from build123d import *

# Parameters (mm, degrees)
BOSS_EXTRUDE1_DEPTH = 6
SKETCH4_R           = 1
CUT_EXTRUDE2_DEPTH  = 230.888016217
SKETCH5_W           = 200
SKETCH5_H           = 20
BOSS_EXTRUDE2_DEPTH = 6
SKETCH6_W           = 184
SKETCH6_H           = 25
CUT_EXTRUDE3_DEPTH  = 230.888016217
SKETCH7_R           = 1
CUT_EXTRUDE4_DEPTH  = 6
BOSS_EXTRUDE3_DEPTH = 6
SKETCH9_R           = 1
CUT_EXTRUDE5_DEPTH  = 245.02561341
SKETCH10_W          = 15
SKETCH10_H          = 143.586884574
BOSS_EXTRUDE4_DEPTH = 6
SKETCH11_R          = 1
CUT_EXTRUDE6_DEPTH  = 245.02561341


with BuildPart() as part:
    # Sketch2 → Boss-Extrude1 (new body)
    with BuildSketch(Plane(origin=(0, 0, 0), x_dir=(1, 0, 0), z_dir=(0, 1, 0))):
        with BuildLine():
            Line((-100, -128.086884574), (-100, 35.5))
            Line((-100, 35.5), (100, 35.5))
            Line((100, 35.5), (100, -128.086884574))
            ThreePointArc((100, -128.086884574), (0, 162.5), (-100, -128.086884574))
        make_face()
    extrude(amount=BOSS_EXTRUDE1_DEPTH)

    # Sketch4 → Cut-Extrude2 (cut, through all)
    with BuildSketch(Plane(origin=(0, 6, 0), x_dir=(1, 0, 0), z_dir=(0, 1, 0))):
        with Locations(Location((119.15, -101.158131161, 0), (0, 0, 270))):
            Circle(SKETCH4_R)
        with Locations(Location((87.75, 86.5, 0), (0, 0, 270))):
            Circle(SKETCH4_R)
        with Locations(Location((152, 23.589123318, 0), (0, 0, 270))):
            Circle(SKETCH4_R)
        with Locations(Location((-87.75, 86.5, 0), (0, 0, 90))):
            Circle(SKETCH4_R)
        with Locations(Location((99, 36.6, 0), (0, 0, 270))):
            Circle(SKETCH4_R)
        with Locations(Location((-99, 36.6, 0), (0, 0, 90))):
            Circle(SKETCH4_R)
        with Locations(Location((-152, 23.589123318, 0), (0, 0, 90))):
            Circle(SKETCH4_R)
        with Locations(Location((-119.15, -101.158131161, 0), (0, 0, 90))):
            Circle(SKETCH4_R)
    extrude(amount=-CUT_EXTRUDE2_DEPTH, mode=Mode.SUBTRACT)

    # Sketch5 → Boss-Extrude2 (add)
    with BuildSketch(Plane(origin=(0, 6, 0), x_dir=(1, 0, 0), z_dir=(0, 1, 0))):
        with Locations((0, -118.086884574)):
            Rectangle(SKETCH5_W, SKETCH5_H)
    extrude(amount=-BOSS_EXTRUDE2_DEPTH)

    # Sketch6 → Cut-Extrude3 (cut, through all)
    with BuildSketch(Plane(origin=(0, 6, 0), x_dir=(1, 0, 0), z_dir=(0, 1, 0))):
        with Locations((0, 48)):
            Rectangle(SKETCH6_W, SKETCH6_H)
    extrude(amount=-CUT_EXTRUDE3_DEPTH, mode=Mode.SUBTRACT)

    # Sketch7 → Cut-Extrude4 (cut)
    with BuildSketch(Plane(origin=(0, 6, 0), x_dir=(1, 0, 0), z_dir=(0, 1, 0))):
        with Locations(Location((-75, 72.8, 0), (0, 0, 270))):
            Circle(SKETCH7_R)
        with Locations(Location((-75, 109.4, 0), (0, 0, 270))):
            Circle(SKETCH7_R)
        with Locations(Location((75, 109.4, 0), (0, 0, 90))):
            Circle(SKETCH7_R)
        with Locations(Location((75, 72.8, 0), (0, 0, 90))):
            Circle(SKETCH7_R)
    extrude(amount=-CUT_EXTRUDE4_DEPTH, mode=Mode.SUBTRACT)

    # Sketch8 → Boss-Extrude3 (add, through all)
    with BuildSketch(Plane(origin=(0, 6, 0), x_dir=(1, 0, 0), z_dir=(0, 1, 0))):
        with BuildLine():
            Line((-100, -128.086884574), (-115.542200083, -128.086884574))
            ThreePointArc((-115.542200083, -128.086884574), (0, 172.5), (115.542200083, -128.086884574))
            Line((115.542200083, -128.086884574), (100, -128.086884574))
            ThreePointArc((100, -128.086884574), (0, 162.5), (-100, -128.086884574))
        make_face()
    extrude(amount=-BOSS_EXTRUDE3_DEPTH)

    # Sketch9 → Cut-Extrude5 (cut, through all)
    with BuildSketch(Plane(origin=(0, 6, 0), x_dir=(1, 0, 0), z_dir=(0, 1, 0))):
        with Locations(Location((0, 167.5, 0), (0, 0, 270))):
            Circle(SKETCH9_R)
        with Locations(Location((83.75, 145.059255134, 0), (0, 0, 270))):
            Circle(SKETCH9_R)
        with Locations(Location((145.059255134, 83.75, 0), (0, 0, 270))):
            Circle(SKETCH9_R)
        with Locations(Location((167.5, 0, 0), (0, 0, 270))):
            Circle(SKETCH9_R)
        with Locations(Location((145.059255134, -83.75, 0), (0, 0, 270))):
            Circle(SKETCH9_R)
        with Locations((83.75, -145.059255134)):
            Circle(SKETCH9_R)
        with Locations((0, -167.5)):
            Circle(SKETCH9_R)
        with Locations((-83.75, -145.059255134)):
            Circle(SKETCH9_R)
        with Locations(Location((-145.059255134, -83.75, 0), (0, 0, 270))):
            Circle(SKETCH9_R)
        with Locations(Location((-167.5, 0, 0), (0, 0, 270))):
            Circle(SKETCH9_R)
        with Locations(Location((-145.059255134, 83.75, 0), (0, 0, 270))):
            Circle(SKETCH9_R)
        with Locations(Location((-83.75, 145.059255134, 0), (0, 0, 270))):
            Circle(SKETCH9_R)
    extrude(amount=-CUT_EXTRUDE5_DEPTH, mode=Mode.SUBTRACT)

    # Sketch10 → Boss-Extrude4 (add, through all)
    with BuildSketch(Plane(origin=(0, 6, 0), x_dir=(1, 0, 0), z_dir=(0, 1, 0))):
        with Locations((-92.5, -36.293442287)):
            Rectangle(SKETCH10_W, SKETCH10_H)
        with Locations((92.5, -36.293442287)):
            Rectangle(SKETCH10_W, SKETCH10_H)
    extrude(amount=-BOSS_EXTRUDE4_DEPTH)

    # Sketch11 → Cut-Extrude6 (cut, through all)
    with BuildSketch(Plane(origin=(0, 6, 0), x_dir=(1, 0, 0), z_dir=(0, 1, 0))):
        with Locations(Location((-90, -118.086884574, 0), (0, 0, 270))):
            Circle(SKETCH11_R)
        with Locations(Location((0, -118.086884574, 0), (0, 0, 270))):
            Circle(SKETCH11_R)
        with Locations(Location((90, -118.086884574, 0), (0, 0, 270))):
            Circle(SKETCH11_R)
        with Locations(Location((-90, 25.5, 0), (0, 0, 270))):
            Circle(SKETCH11_R)
        with Locations(Location((-90, -41.293442287, 0), (0, 0, 270))):
            Circle(SKETCH11_R)
        with Locations(Location((90, -41.293442287, 0), (0, 0, 90))):
            Circle(SKETCH11_R)
        with Locations(Location((90, 25.5, 0), (0, 0, 90))):
            Circle(SKETCH11_R)
    extrude(amount=-CUT_EXTRUDE6_DEPTH, mode=Mode.SUBTRACT)


solid = part.part
Geometry: final body of the model. Coordinates: model frame, mm. Coordinates: 2 decimals unless noted, no trailing zeros. Order: outer loops, then holes, each group sorted by start corner. A loop starts at its lowest first (then second) coordinate and runs counter-clockwise, first axis right, second up.
(1) Section query B-B (z = -52.5). Return the cut outline in (x, y).
(2) Section query C-C (y = 1.5). State how many separate pieces and enclosed holes the cut face has, plus the area to 3 significant figures.
(3) First-contact query: pin 1 (1.8 mm diameter, centred on x = 11.5, y = 3, fed in from -Z); pin 2 (3 mm diameter, centred on y = 3, z = 70.5, fed in from +X); pin 3 (1.8 mm diameter, centred on x = -90, z = -25.5, fed in from -Y); pin 4 (2 mm diameter, centred on x = -92, y = 5, fed in from -Z). Flat tips, straight axial feed; report the tip coordinate or a pass-through.
(4) Draft query along Y for faces 1 (the face through (-2, 0, -91)), 2 (the face through (-2, 6, -91)), 3 (the face through (-5.813, 3.042, -172.402)). Return one class per face: pulls with the +Y half, pulls with the -Y half, needs draft (parallel to the pull), parting line crosses it, or undercut.
(5) Material intervals for probe 1 along X at (y, z) = (1.5, -36.6); probe 2 along X at (y, z) = (3.55, 40.5); probe 3 along Z at (x, y) = (-90, 4.75), sorted ascending.
(6) Section query A-A (x = -45). Return the cut outline in (y, z).
Solution:
1. outline: (-164.32, 0) - (-92, 0) - (-92, 6) - (-164.32, 6) - close; (92, 0) - (164.32, 0) - (164.32, 6) - (92, 6) - close
2. separate pieces: 1
2. enclosed holes: 29
2. area: 57,300 mm2
3. pin 1: stops at z = -172.17
3. pin 2: stops at x = 158.1
3. pin 3: passes through
3. pin 4: stops at z = -146.54
4. face 1: pulls with the -Y half
4. face 2: pulls with the +Y half
4. face 3: needs draft
5. probe 1: x = -168.57 to -100, -98 to -92, 92 to 98, 100 to 168.57
5. probe 2: x = -167.68 to -90.61, -89.39 to -85, 85 to 89.39, 90.61 to 167.68
5. probe 3: z = -147.16 to -60.5, -35.5 to -26.5, -24.5 to 40.29, 42.29 to 117.09, 119.09 to 128.09
6. outline: (0, -166.53) - (6, -166.53) - (6, -60.5) - (0, -60.5) - close; (0, 108.09) - (6, 108.09) - (6, 128.09) - (0, 128.09) - close
